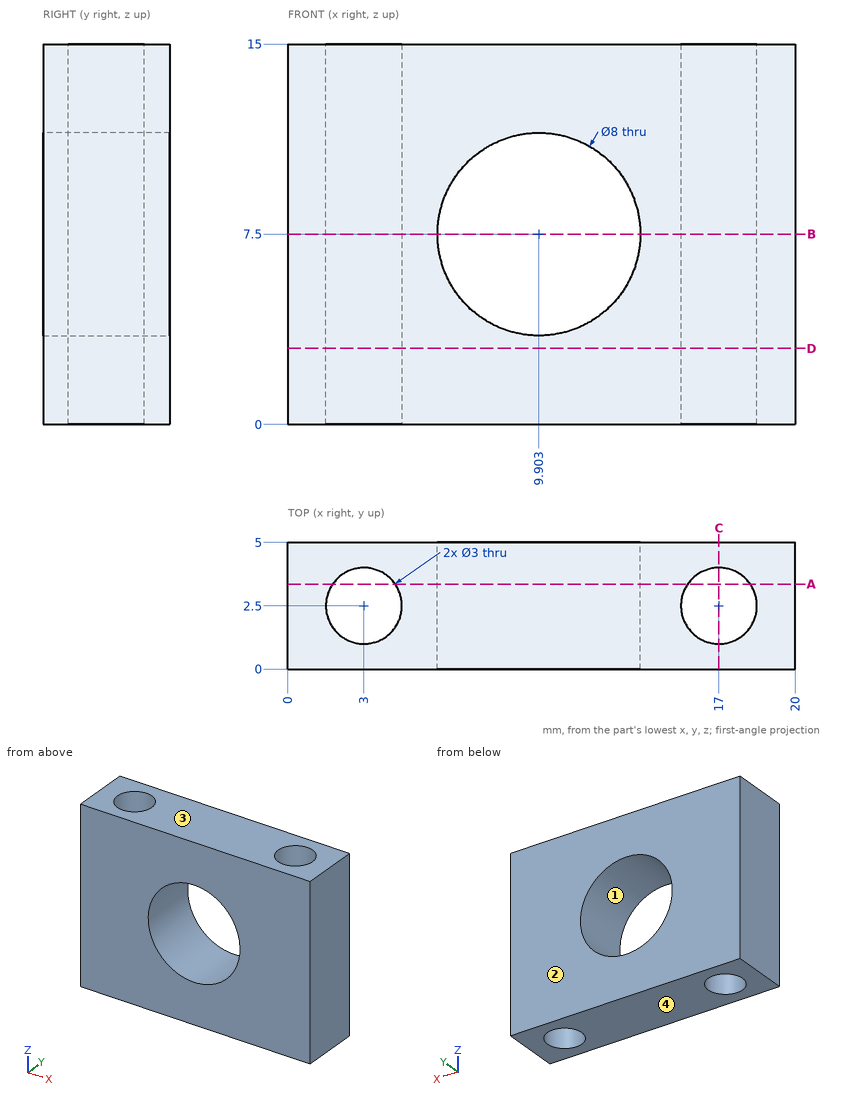
For this review, use the dimensioned drawing (mm, ordinates from the lowest corner) and the shaded views. Round coordinates to 2 decimals unless told otherwise and drop trailing zeros. Write each loop counter-clockwise with the first axis right and the second up, starting at its lowest first coordinate (ties: lowest second). Pieces come first, ordered by that corner, then holes. Notation, with made-up numbers: (28, 33) - (86, 33) arc R21 cw to (86, 62) - close; hole circle Ø3 at (76.5, 78). An arc over 180 degrees is marked (long way). Use CSV: the item, a comma, the result in double quotes.
1) Add section D-D on z = 3. Write out the cut boundary in (x, y).
Conclusion:
outline,"(0, 0) - (20, 0) - (20, 5) - (0, 5) - close; hole circle Ø3 at (3, 2.5); hole circle Ø3 at (17, 2.5)"
2) Add section B-B on z = 7.5. Write out the cut boundary in (x, y).
Conclusion:
outline,"(0, 0) - (5.9, 0) - (5.9, 5) - (0, 5) - close; (13.9, 0) - (20, 0) - (20, 5) - (13.9, 5) - close; hole circle Ø3 at (3, 2.5); hole circle Ø3 at (17, 2.5)"
3) Add section C-C on x = 17. Write out the cut boundary in (y, z), and give its area (3 significant figures).
Conclusion:
outline,"(0, 0) - (1, 0) - (1, 15) - (0, 15) - close; (4, 0) - (5, 0) - (5, 15) - (4, 15) - close"
area,"30.0 mm^2"
4) The part is to be moulded in two halves that separate along Z. For the marked faces 1, 2, 3 and 4, say which applies: pulls with the +Z half, pulls with the -Z half, needs draft (parallel to the pull), parting line crosses it, or undercut.
Conclusion:
face 1,"undercut"
face 2,"needs draft"
face 3,"pulls with the +Z half"
face 4,"pulls with the -Z half"
5) Wall thickness on line 1 along Y through (x, z) = (17, 3.5); line 2 along X through (y, z) = (1.65, 7.5) (1 decimal); line 3 along X through (y, z) = (3, 2.75) (1 decimal): over which ranges is each line inside the solid? List them lowest first. Write a range as from..to.
Conclusion:
line 1,"y = 0..1, 4..5"
line 2,"x = 0..1.8, 4.2..5.9, 13.9..15.8, 18.2..20"
line 3,"x = 0..1.6, 4.4..15.6, 18.4..20"
6) Add section A-A on y = 3.35. Write out the cut boundary in (x, z).
Conclusion:
outline,"(0, 0) - (1.76, 0) - (1.76, 15) - (0, 15) - close; (4.24, 0) - (15.76, 0) - (15.76, 15) - (4.24, 15) - close; (18.24, 0) - (20, 0) - (20, 15) - (18.24, 15) - close; hole circle Ø8 at (9.9, 7.5)"
